```python
from build123d import *

# Parameters (mm, degrees)
ESQUISSE2_R             = 110
BOSS_EXTRU_1_DEPTH      = 2
ESQUISSE7_R             = 2
ESQUISSE7_R_2           = 1.991144914
ENL_V_MAT_EXTRU_7_DEPTH = 2


with BuildPart() as part:
    # Esquisse2 → Boss.-Extru.1 (new body)
    with BuildSketch(Plane.XY):
        Circle(ESQUISSE2_R)
    extrude(amount=BOSS_EXTRU_1_DEPTH)

    # Esquisse7 → Enlèv. mat.-Extru.7 (cut)
    with BuildSketch(Plane(origin=(0, 0, 0), x_dir=(-1, 0, 0), z_dir=(0, 0, -1))):
        with Locations((-15, 98.868599666)):
            Circle(ESQUISSE7_R)
        with Locations((15, 98.868599666)):
            Circle(ESQUISSE7_R_2)
        with Locations((69.377054927, -39.718437198)):
            Circle(ESQUISSE7_R)
        with Locations((93.122718948, -36.443918776)):
            Circle(ESQUISSE7_R)
        with Locations((78.122718948, -62.42468089)):
            Circle(ESQUISSE7_R_2)
        with Locations((-68.990680451, -39.941510605)):
            Circle(ESQUISSE7_R)
        with Locations((-78.122718948, -62.42468089)):
            Circle(ESQUISSE7_R)
        with Locations((-93.122718948, -36.443918776)):
            Circle(ESQUISSE7_R_2)
        with Locations((0, 80)):
            Circle(ESQUISSE7_R)
    extrude(amount=-ENL_V_MAT_EXTRU_7_DEPTH, mode=Mode.SUBTRACT)


solid = part.part
```
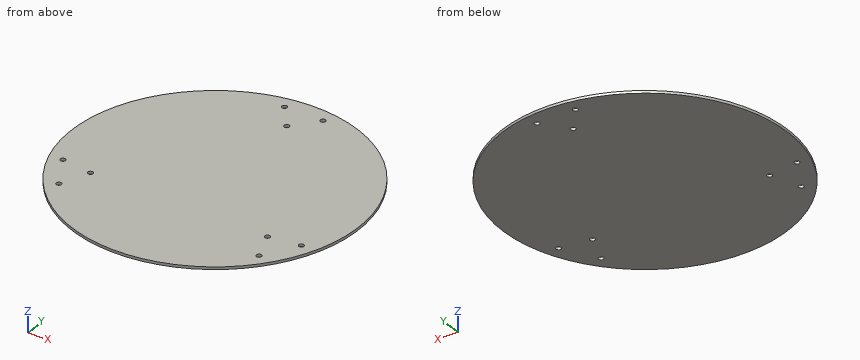
Source: CAD feature listing. Evaluate the final solid. Frame: model axes, mm. Round coordinates to 2 decimals unless told otherwise and drop trailing zeros. Write each loop counter-clockwise with the first axis right and the second up, starting at its lowest first coordinate (ties: lowest second). Pieces come first, ordered by that corner, then holes. Notation, with made-up numbers: M -38,58 L 3,58 A21 ccw 3,79 Z; hole C 3,-5.5 d1. An arc over 180 degrees is marked long. Answer as a JSON object with one key per item and string values. Group by question number.
(1) Section query C-C on x = 32.5. Output: boundary loops of the cut face in (y, z), then the cut area to 3 significant figures.
(2) First-contact query: pin 1 (1 mm diameter, centred on y = 56.5, z = 1.5, fed in from +X). Flat tip, straight axial feed; report the tip coordinate or a pass-through.
(3) Ray query, line 1 (Y direction, x = -15, z = 0.7); line 2 (X direction, y = -38.5, z = 0.1); line 3 (X direction, y = 1.5, z = 1.9). Return the intervals inside material, ascending. Write a range as [from, to].
(4) Section query A-A on z = 1.15. State how many separate pieces and enclosed holes the cut face has, then the cut area to 3 significant figures.
(5) Section query B-B on x = -64.5. Output: boundary loops of the cut face in (y, z).
Computed values:
{
 "1": {"outline": "M -105.09,0 L 105.09,0 L 105.09,2 L -105.09,2 Z", "area": "420 mm^2"},
 "2": {"pin 1": "x = 94.68"},
 "3": {"line 1": "[-108.97, 96.88], [100.86, 108.97]", "line 2": "[-103.04, -70.96], [-67.79, 67.6], [70.38, 103.04]", "line 3": "[-109.99, 109.99]"},
 "4": {"separate pieces": "1", "enclosed holes": "9", "area": "37,900 mm^2"},
 "5": {"outline": "M -89.11,0 L 89.11,0 L 89.11,2 L -89.11,2 Z"}
}
